CAD build for the part. Positions are in the model's coordinates, mm. Face numbers are marked on the shaded views. A direction names the side the tool comes from. Give positions to 0.01 mm unless a question says otherwise; leave off trailing zeros. Write each loop counter-clockwise with the first axis right and the second up, starting at its lowest first coordinate (ties: lowest second). Pieces come first, ordered by that corner, then holes. Notation, with made-up numbers: M -18.75,-15 L -13.75,-15 A10 cw -13.75,-6 Z; hole C 16.25,-3.5 d11. An arc over 180 degrees is marked long. One line per question, with ' | ' between items. Start each with the question number.
1. Which spindle directions (+Z, -Z, +X, -X, +Y, -Y) get a long thin tool onto all of the face, cutting with end or side? Do the marked faces 1 and 2. Say none if no direction does.
2. Flat gauge pins, fed straight in: pin 1 (0.6 mm diameter, centred on x = 244.5, z = 1.5, fed in from +Y); pin 2 (3 mm diameter, centred on x = 216, z = 15.5, fed in from +Y); pin 3 (1 mm diameter, centred on x = 348, y = 41, fed in from +Z); pin 4 (5 mm diameter, centred on y = 10, z = 5.5, fed in from +X). Where does each tip first touch, or does it go through?
3. Wall check: L1, parallel to Y at x = 374.5, z = 14; L2, parallel to Y at x = 330, z = 1.5. Give the ranges that are in metal, low to high.
4. Cut at C-C, the plane z = 10.5. Write the cut outline in (x, y).
5. Cut at B-B, the plane x = 287.5. Write the cut outline in (y, z), then the cut area to 3 significant figures.
6. Cut at A-A, the plane y = 36. Write the cut outline in (x, z), then the cut area to 3 significant figures.
Autodesk Inventor part; units mm, degrees
ref_plane "YZ Plane" through (0, 0, 0) normal (1, 0, 0) x (0, 1, 0)
ref_plane "XZ Plane" through (0, 0, 0) normal (0, 1, 0) x (-1, 0, 0)
ref_plane "XY Plane" through (0, 0, 0) normal (0, 0, 1) x (1, 0, 0)
sketch "Sketch1" plane through (0, 0, 0) normal (0, 0, 1) x (1, 0, 0)
  line L0 (-490, 52) -> (490, 52)
  line L1 (490, 52) -> (490, 0)
  line L2 (490, 0) -> (-490, 0)
  line L3 (-490, 0) -> (-490, 52)
  point P0 (0, 0)
  point P1 (0, 0)
  dimension "d0" = 980
  dimension "d1" = 52
extrude "Plate1" add sketch "Sketch1" along normal blind 2
sketch "Sketch2" plane through (490, 2, 0) normal (0, -1, 0) x (1, 0, 0)
  line L0 (-980, 0) -> (0, 0)
  line L1 (0, 0) -> (0, 20)
  line L2 (0, 20) -> (-980, 20)
  line L3 (-980, 20) -> (-980, 0)
edge flange "Flange1" height 20 angle 90 thickness 2 bend radius 2.75 thickness toward (0, -1, 0) relief round relief width 2 relief depth 1 edges at (0, 0, 2) wall of the first edge with corners at (-490, 2, 0) (490, 2, 0) (490, 2, 20) (-490, 2, 20)
bend "Bend1"
corner "Corner1"
sketch "Sketch11" plane through (0, 0, 0) normal (0, 0, 1) x (1, 0, 0)
  line L0 (-490, 52) -> (490, 52)
  circle A0 centre (0, 52) radius 30
  line L1 (-490, 0) -> (490, 0)
  line L2 (246.05, 0) -> (243.95, 0)
  line L3 (243.95, 0) -> (243.95, 29)
  line L4 (243.95, 29) -> (246.05, 29)
  line L5 (246.05, 29) -> (246.05, 0)
  line L6 (-243.95, 0) -> (-246.05, 0)
  line L7 (-246.05, 0) -> (-246.05, 29) construction
  line L8 (-246.05, 29) -> (-243.95, 29) construction
  line L9 (-243.95, 29) -> (-243.95, 0) construction
  line L10 (0, 52) -> (0, 0)
  line L11 (246.05, 29) -> (246.05, 52)
  line L12 (243.95, 29) -> (243.95, 52)
  line L13 (-243.95, 29) -> (-243.95, 52) construction
  line L14 (-246.05, 29) -> (-246.05, 52) construction
  line L15 (-490, 0) -> (-490, 52)
  circle A1 centre (490, 52) radius 30
  line L16 (490, 52) -> (490, 0)
  point P0 (30, 52)
  point P1 (-30, 52)
  point P2 (-245, 29)
  point P3 (245, 29)
  point P4 (490, 22)
  point P5 (460, 52)
  point P6 (0, 22)
  dimension "d44" = 60
  dimension "d47" = 2.1
  dimension "d49" = 490
  dimension "d50" = 29
extrude "Extrusion4" cut sketch "Sketch11" along normal through all both and the other way through all contours L10 A0 L0 | A0 L10 L1 L15 L0 | L0 L11 L4 L12 picked at (-19.7493, 49.7748)
sketch "Sketch9" plane through (0, 0, 2) normal (0, 0, 1) x (1, 0, 0)
  line L0 (456.3279, 23.6801) -> (456.3279, 11.6801) construction
  line L1 (456.3279, 11.6801) -> (256.3279, 11.6801) construction
  line L2 (256.3279, 11.6801) -> (256.3279, 23.6801) construction
  line L3 (256.3279, 23.6801) -> (456.3279, 23.6801) construction
  line L4 (-490, 52) -> (490, 52)
  point P0 (0, 0)
  point P1 (1, 52)
  dimension "d38" = 200
  dimension "d39" = 12
mark "Mark3"
equation "\"d1\" = СПИНА_Стрингер_1_высота"
equation "\"d2\" = Thickness"
equation "\"d3\" = BendReliefWidth"
equation "\"d4\" = BendReliefDepth"
equation "\"d5\" = MinimumRemnant"
equation "\"d6\" = TransitionRadius"
equation "\"d9\" = BendRadius"
equation "\"d10\" = CornerReliefSize"
equation "\"d11\" = GapSize"
equation "\"d12\" = JacobiRadiusSize"
equation "\"BendReliefWidth\" = Thickness"
equation "\"BendReliefDepth\" = 0.5 * Thickness"
equation "\"CornerReliefSize\" = 4 * Thickness"
equation "\"MinimumRemnant\" = 2 * Thickness"
equation "\"TransitionRadius\" = BendRadius"
equation "\"JacobiRadiusSize\" = BendRadius"
equation "\"GapSize\" = Thickness"
properties part number "MSC 204 stringer back ^" material "Stainless Steel"
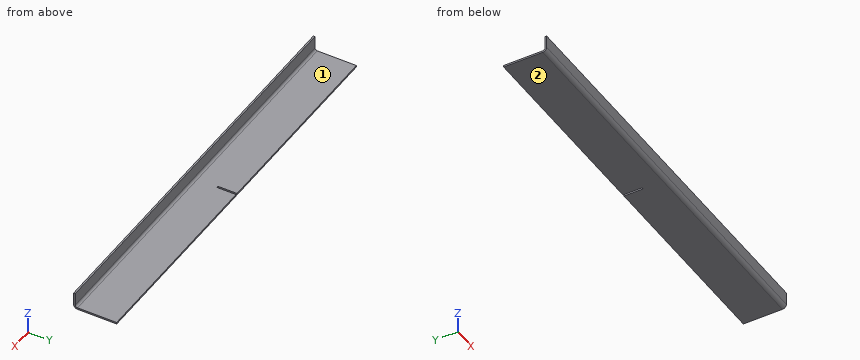
Here are the results:
1) face 1: +Z, +X, -X, +Y | face 2: -Z, +X, -X, +Y, -Y
2) pin 1: y = 29 | pin 2: y = 2 | pin 3: z = 2 | pin 4: through
3) L1: 0 to 2 | L2: 1.29 to 52
4) outline: M 0,0 L 490,0 L 490,2 L 0,2 Z
5) outline: M 0,4.75 A4.75 ccw 4.75,0 L 52,0 L 52,2 L 4.75,2 A2.75 cw 2,4.75 L 2,20 L 0,20 Z | area: 137 mm^2
6) outline: M 0,0 L 243.95,0 L 243.95,2 L 0,2 Z; M 246.05,0 L 490,0 L 490,2 L 246.05,2 Z | area: 976 mm^2
